Here's how the part is built. I have some questions about the finished solid (model axes, mm). Face numbers are marked on the shaded views. A direction names the side the tool comes from. Coordinates: 2 decimals unless noted, no trailing zeros. Order: outer loops, then holes, each group sorted by start corner. A loop starts at its lowest first (then second) coordinate and runs counter-clockwise, first axis right, second up. Notation, with made-up numbers: (-29, 19) - (-24, 19) arc R18 cw to (-24, 42) - close; hole circle Ø4 at (62.25, 77). An arc over 180 degrees is marked (long way). Answer as CSV lines item,"result". Start each with the question number.
Item 1: Imagine slicing it at A-A on y = -34. List the corners of the cut face in (x, z) for me.
Item 2: Imagine slicing it at B-B on x = -25. List the corners of the cut face in (y, z) for me, and give its area (3 significant figures).
Item 3: I'm going to push flat-ended pins straight in: pin 1 (9.5 mm diameter, centred on x = -25, z = 14, fed in from -Y) (1 decimal); pin 2 (1.8 mm diameter, centred on x = -6, z = 7, fed in from +Y); pin 3 (2 mm diameter, centred on x = -0.5, y = 4, fed in from +Z); pin 4 (5.5 mm diameter, centred on x = -27, z = 9.5, fed in from -Y). Where does each tip first touch, or does it pass through?
Item 4: I need wall thicknesses on line 1 (X direction, y = -28, z = 1.5); line 2 (Z direction, x = 25, y = -42); line 3 (Y direction, x = 17, z = 19.5). Which ranges of each line are inside material? Lowest first, please.
Item 5: We'd pull the mould along Z, two halves only. Please class the marked faces 1, 2, 3 and 4: pulls with the +Z half, pulls with the -Z half, needs draft (parallel to the pull), parting line crosses it, or undercut.
Item 6: Imagine slicing it at C-C on z = 6.5. List the corners of the cut face in (x, y) for me, and give its area (3 significant figures).
Item 7: Imagine slicing it at D-D on y = -7. List the corners of the cut face in (x, z) for me.
Item 8: On a 3-axis mill with a long thin cutter (end or side, diameter ignored), from which of +Z, -Z, +X, -X, +Y, -Y can I reach the whole of each face in a straight line? I mean the marked faces 5 and 6. Say none if no direction works.
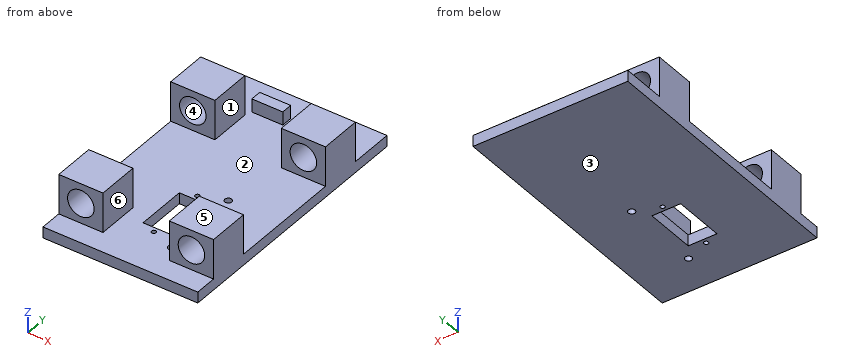
from build123d import *

# Parameters (mm, degrees)
SKETCH1_W           = 70
SKETCH1_H           = 120
BOSS_EXTRUDE1_DEPTH = 5
SKETCH2_W           = 20
SKETCH2_H           = 19
BOSS_EXTRUDE2_DEPTH = 18
SKETCH3_R           = 6
CUT_EXTRUDE1_DEPTH  = 109.415865998
CUT_EXTRUDE2_REACH  = 75.171
SKETCH4_R           = 1
SKETCH4_W           = 13
SKETCH4_H           = 23
SKETCH5_W           = 14
SKETCH5_H           = 5
BOSS_EXTRUDE3_DEPTH = 6
SKETCH6_R           = 1.55
CUT_EXTRUDE3_DEPTH  = 74.17103252


with BuildPart() as part:
    # Sketch1 → Boss-Extrude1 (new body)
    with BuildSketch(Plane.XY):
        Rectangle(SKETCH1_W, SKETCH1_H)
    extrude(amount=BOSS_EXTRUDE1_DEPTH)

    # Sketch2 → Boss-Extrude2 (add)
    with BuildSketch(Plane.XY.offset(5)):
        with Locations((-25, 30.5)):
            Rectangle(SKETCH2_W, SKETCH2_H)
        with Locations((25, 30.5)):
            Rectangle(SKETCH2_W, SKETCH2_H)
        with Locations((-25, -40.5)):
            Rectangle(SKETCH2_W, SKETCH2_H)
        with Locations((25, -40.5)):
            Rectangle(SKETCH2_W, SKETCH2_H)
    extrude(amount=BOSS_EXTRUDE2_DEPTH)

    # Sketch3 → Cut-Extrude1 (cut, through all)
    with BuildSketch(Plane(origin=(0, 40, 0), x_dir=(1, 0, 0), z_dir=(0, 1, 0))):
        with Locations(Location((-25, -14, 0), (0, 0, 180))):
            Circle(SKETCH3_R)
        with Locations(Location((25, -14, 0), (0, 0, 180))):
            Circle(SKETCH3_R)
    extrude(amount=-CUT_EXTRUDE1_DEPTH, mode=Mode.SUBTRACT)

    # Sketch4 → Cut-Extrude2 (cut, up to next)
    with BuildSketch(Plane(origin=(0, 0, 0), x_dir=(-1, 0, 0), z_dir=(0, 0, -1)), mode=Mode.PRIVATE) as cut_extrude2_sk1:
        with Locations((0, -11.2)):
            Circle(SKETCH4_R)
    cut_extrude2_tool1 = extrude(cut_extrude2_sk1.sketch, amount=-CUT_EXTRUDE2_REACH, mode=Mode.PRIVATE) & part.part
    # Sketch4 → Cut-Extrude2 (cut, up to next)
    with BuildSketch(Plane(origin=(0, 0, 0), x_dir=(-1, 0, 0), z_dir=(0, 0, -1)), mode=Mode.PRIVATE) as cut_extrude2_sk2:
        with Locations((0, -38.8)):
            Circle(SKETCH4_R)
    cut_extrude2_tool2 = extrude(cut_extrude2_sk2.sketch, amount=-CUT_EXTRUDE2_REACH, mode=Mode.PRIVATE) & part.part
    # Sketch4 → Cut-Extrude2 (cut, up to next)
    with BuildSketch(Plane(origin=(0, 0, 0), x_dir=(-1, 0, 0), z_dir=(0, 0, -1)), mode=Mode.PRIVATE) as cut_extrude2_sk3:
        with Locations((0, -25)):
            Rectangle(SKETCH4_W, SKETCH4_H)
    cut_extrude2_tool3 = extrude(cut_extrude2_sk3.sketch, amount=-CUT_EXTRUDE2_REACH, mode=Mode.PRIVATE) & part.part
    add(cut_extrude2_tool1.solids().sort_by_distance((0, -11.2, 0))[0], mode=Mode.SUBTRACT)
    add(cut_extrude2_tool2.solids().sort_by_distance((0, -38.8, 0))[0], mode=Mode.SUBTRACT)
    add(cut_extrude2_tool3.solids().sort_by_distance((0, -25, 0))[0], mode=Mode.SUBTRACT)

    # Sketch5 → Boss-Extrude3 (add)
    with BuildSketch(Plane.XY.offset(5)):
        with Locations((-7, 45.5)):
            Rectangle(SKETCH5_W, SKETCH5_H)
    extrude(amount=BOSS_EXTRUDE3_DEPTH)

    # Sketch6 → Cut-Extrude3 (cut, through all)
    with BuildSketch(Plane(origin=(0, 0, 0), x_dir=(-1, 0, 0), z_dir=(0, 0, -1))):
        with Locations((-11, -7)):
            Circle(SKETCH6_R)
        with Locations((-11, -43)):
            Circle(SKETCH6_R)
    extrude(amount=-CUT_EXTRUDE3_DEPTH, mode=Mode.SUBTRACT)


solid = part.part
Responses:
1,outline,"(-35, 0) - (-6.5, 0) - (-6.5, 5) - (-15, 5) - (-15, 23) - (-35, 23) - close; (6.5, 0) - (35, 0) - (35, 23) - (15, 23) - (15, 5) - (6.5, 5) - close; hole circle Ø12 at (-25, 14); hole circle Ø12 at (25, 14)"
2,outline,"(-60, 0) - (60, 0) - (60, 5) - (40, 5) - (40, 8) - (21, 8) - (21, 5) - (-31, 5) - (-31, 8) - (-50, 8) - (-50, 5) - (-60, 5) - close; (-50, 20) - (-31, 20) - (-31, 23) - (-50, 23) - close; (21, 20) - (40, 20) - (40, 23) - (21, 23) - close"
2,area,"828 mm^2"
3,pin 1,"passes through"
3,pin 2,"stops at y = 48"
3,pin 3,"stops at z = 5"
3,pin 4,"stops at y = -50"
4,line 1,"x = -35 to -6.5, 6.5 to 35"
4,line 2,"z = 0 to 8, 20 to 23"
4,line 3,"y = -50 to -31, 21 to 40"
5,face 1,"needs draft"
5,face 2,"pulls with the +Z half"
5,face 3,"pulls with the -Z half"
5,face 4,"undercut"
6,outline,"(-35, -50) - (-15, -50) - (-15, -31) - (-35, -31) - close; (-35, 21) - (-15, 21) - (-15, 40) - (-35, 40) - close; (-14, 43) - (0, 43) - (0, 48) - (-14, 48) - close; (15, -50) - (35, -50) - (35, -31) - (15, -31) - close; (15, 21) - (35, 21) - (35, 40) - (15, 40) - close"
6,area,"1,590 mm^2"
7,outline,"(-35, 0) - (9.45, 0) - (9.45, 5) - (-35, 5) - close; (12.55, 0) - (35, 0) - (35, 5) - (12.55, 5) - close"
8,face 5,"+Z, +X, -X, +Y, -Y"
8,face 6,"+Z, +Y, -Y"
